The listing builds one solid part. Answer for the finished solid, in the listing's coordinates (mm). A direction names the side the tool comes from. Coordinates: 2 decimals unless noted, no trailing zeros. Loops run counter-clockwise (first coordinate to the right, second up) from the corner with the lowest first, then second, coordinate; pieces in that order, holes last. Notation, with made-up numbers: (14, 17) - (65, 17) arc R25 cw to (65, 51) - close; hole circle Ø5 at (17.25, 43.5). An arc over 180 degrees is marked (long way). Put each result on its own line as item: value.
```python
from build123d import *

# Parameters (mm, degrees)
SKETCH1_R           = 140
BOSS_EXTRUDE1_DEPTH = 3
CUT_EXTRUDE3_REACH  = 200.013
SKETCH19_R          = 1.5
CUT_EXTRUDE10_REACH = 200.013
SKETCH25_R          = 1.5
CUT_EXTRUDE4_REACH  = 200.013
FILLET2_R           = 10
SKETCH26_R          = 1.5
CUT_EXTRUDE11_DEPTH = 3
FILLET6_R           = 3
FILLET7_R           = 1


with BuildPart() as part:
    # Sketch1 → Boss-Extrude1 (new body)
    with BuildSketch(Plane(origin=(0, 0, 0), x_dir=(1, 0, 0), z_dir=(0, 1, 0))):
        with Locations(Location((0, 0, 0), (0, 0, 270))):
            Circle(SKETCH1_R)
    extrude(amount=BOSS_EXTRUDE1_DEPTH)

    # Sketch19 → Cut-Extrude3 (cut, up to next)
    with BuildSketch(Plane(origin=(0, 3, 0), x_dir=(1, 0, 0), z_dir=(0, 1, 0)), mode=Mode.PRIVATE) as cut_extrude3_sk1:
        with Locations(Location((-89.09545443, -67.882250994, 0), (0, 0, 270))):
            Circle(SKETCH19_R)
    cut_extrude3_tool1 = extrude(cut_extrude3_sk1.sketch, amount=-CUT_EXTRUDE3_REACH, mode=Mode.PRIVATE) & part.part
    # Sketch19 → Cut-Extrude3 (cut, up to next)
    with BuildSketch(Plane(origin=(0, 3, 0), x_dir=(1, 0, 0), z_dir=(0, 1, 0)), mode=Mode.PRIVATE) as cut_extrude3_sk2:
        with Locations(Location((-89.09545443, 67.882250994, 0), (0, 0, 270))):
            Circle(SKETCH19_R)
    cut_extrude3_tool2 = extrude(cut_extrude3_sk2.sketch, amount=-CUT_EXTRUDE3_REACH, mode=Mode.PRIVATE) & part.part
    # Sketch19 → Cut-Extrude3 (cut, up to next)
    with BuildSketch(Plane(origin=(0, 3, 0), x_dir=(1, 0, 0), z_dir=(0, 1, 0)), mode=Mode.PRIVATE) as cut_extrude3_sk3:
        with Locations(Location((89.09545443, 67.882250994, 0), (0, 0, 270))):
            Circle(SKETCH19_R)
    cut_extrude3_tool3 = extrude(cut_extrude3_sk3.sketch, amount=-CUT_EXTRUDE3_REACH, mode=Mode.PRIVATE) & part.part
    # Sketch19 → Cut-Extrude3 (cut, up to next)
    with BuildSketch(Plane(origin=(0, 3, 0), x_dir=(1, 0, 0), z_dir=(0, 1, 0)), mode=Mode.PRIVATE) as cut_extrude3_sk4:
        with Locations(Location((89.09545443, -67.882250994, 0), (0, 0, 270))):
            Circle(SKETCH19_R)
    cut_extrude3_tool4 = extrude(cut_extrude3_sk4.sketch, amount=-CUT_EXTRUDE3_REACH, mode=Mode.PRIVATE) & part.part
    # Sketch19 → Cut-Extrude3 (cut, up to next)
    with BuildSketch(Plane(origin=(0, 3, 0), x_dir=(1, 0, 0), z_dir=(0, 1, 0)), mode=Mode.PRIVATE) as cut_extrude3_sk5:
        with Locations(Location((-67.882250994, 89.09545443, 0), (0, 0, 270))):
            Circle(SKETCH19_R)
    cut_extrude3_tool5 = extrude(cut_extrude3_sk5.sketch, amount=-CUT_EXTRUDE3_REACH, mode=Mode.PRIVATE) & part.part
    # Sketch19 → Cut-Extrude3 (cut, up to next)
    with BuildSketch(Plane(origin=(0, 3, 0), x_dir=(1, 0, 0), z_dir=(0, 1, 0)), mode=Mode.PRIVATE) as cut_extrude3_sk6:
        with Locations(Location((67.882250994, 89.09545443, 0), (0, 0, 270))):
            Circle(SKETCH19_R)
    cut_extrude3_tool6 = extrude(cut_extrude3_sk6.sketch, amount=-CUT_EXTRUDE3_REACH, mode=Mode.PRIVATE) & part.part
    # Sketch19 → Cut-Extrude3 (cut, up to next)
    with BuildSketch(Plane(origin=(0, 3, 0), x_dir=(1, 0, 0), z_dir=(0, 1, 0)), mode=Mode.PRIVATE) as cut_extrude3_sk7:
        with Locations(Location((67.882250994, -89.09545443, 0), (0, 0, 270))):
            Circle(SKETCH19_R)
    cut_extrude3_tool7 = extrude(cut_extrude3_sk7.sketch, amount=-CUT_EXTRUDE3_REACH, mode=Mode.PRIVATE) & part.part
    # Sketch19 → Cut-Extrude3 (cut, up to next)
    with BuildSketch(Plane(origin=(0, 3, 0), x_dir=(1, 0, 0), z_dir=(0, 1, 0)), mode=Mode.PRIVATE) as cut_extrude3_sk8:
        with Locations(Location((-67.882250994, -89.09545443, 0), (0, 0, 270))):
            Circle(SKETCH19_R)
    cut_extrude3_tool8 = extrude(cut_extrude3_sk8.sketch, amount=-CUT_EXTRUDE3_REACH, mode=Mode.PRIVATE) & part.part
    add(cut_extrude3_tool1.solids().sort_by_distance((-89.095454, 3, 67.882251))[0], mode=Mode.SUBTRACT)
    add(cut_extrude3_tool2.solids().sort_by_distance((-89.095454, 3, -67.882251))[0], mode=Mode.SUBTRACT)
    add(cut_extrude3_tool3.solids().sort_by_distance((89.095454, 3, -67.882251))[0], mode=Mode.SUBTRACT)
    add(cut_extrude3_tool4.solids().sort_by_distance((89.095454, 3, 67.882251))[0], mode=Mode.SUBTRACT)
    add(cut_extrude3_tool5.solids().sort_by_distance((-67.882251, 3, -89.095454))[0], mode=Mode.SUBTRACT)
    add(cut_extrude3_tool6.solids().sort_by_distance((67.882251, 3, -89.095454))[0], mode=Mode.SUBTRACT)
    add(cut_extrude3_tool7.solids().sort_by_distance((67.882251, 3, 89.095454))[0], mode=Mode.SUBTRACT)
    add(cut_extrude3_tool8.solids().sort_by_distance((-67.882251, 3, 89.095454))[0], mode=Mode.SUBTRACT)

    # Sketch25 → Cut-Extrude10 (cut, up to next)
    with BuildSketch(Plane(origin=(0, 3, 0), x_dir=(1, 0, 0), z_dir=(0, 1, 0)), mode=Mode.PRIVATE) as cut_extrude10_sk1:
        with Locations(Location((-124, 50, 0), (0, 0, 270))):
            Circle(SKETCH25_R)
    cut_extrude10_tool1 = extrude(cut_extrude10_sk1.sketch, amount=-CUT_EXTRUDE10_REACH, mode=Mode.PRIVATE) & part.part
    # Sketch25 → Cut-Extrude10 (cut, up to next)
    with BuildSketch(Plane(origin=(0, 3, 0), x_dir=(1, 0, 0), z_dir=(0, 1, 0)), mode=Mode.PRIVATE) as cut_extrude10_sk2:
        with Locations(Location((-124, -50, 0), (0, 0, 270))):
            Circle(SKETCH25_R)
    cut_extrude10_tool2 = extrude(cut_extrude10_sk2.sketch, amount=-CUT_EXTRUDE10_REACH, mode=Mode.PRIVATE) & part.part
    add(cut_extrude10_tool1.solids().sort_by_distance((-124, 3, -50))[0], mode=Mode.SUBTRACT)
    add(cut_extrude10_tool2.solids().sort_by_distance((-124, 3, 50))[0], mode=Mode.SUBTRACT)

    # Sketch20 → Cut-Extrude4 (cut, up to next)
    with BuildSketch(Plane(origin=(0, 3, 0), x_dir=(1, 0, 0), z_dir=(0, 1, 0)), mode=Mode.PRIVATE) as cut_extrude4_sk1:
        Polygon((-553.578520829, 601.645168987), (-72, 120.066648158), (-50, 98.066648158), (50, 98.066648158), (72, 120.066648158), (553.578520829, 601.645168987), (553.578520829, 1963.754919995), (-553.578520829, 1963.754919995), align=None)
    cut_extrude4_tool1 = extrude(cut_extrude4_sk1.sketch, amount=-CUT_EXTRUDE4_REACH, mode=Mode.PRIVATE) & part.part
    add(cut_extrude4_tool1.solids().sort_by_distance((0, 3, -1137.970098))[0], mode=Mode.SUBTRACT)

    # Fillet2
    fillet2_edges = [part.edges().sort_by_distance(p)[0] for p in [
        (50, 1.5, -98.066648158),
        (-50, 1.5, -98.066648158),
    ]]
    fillet(fillet2_edges, radius=FILLET2_R)

    # Sketch26 → Cut-Extrude11 (cut)
    # profile 1 of 7: a face of its own
    with BuildSketch(Plane(origin=(0, 3, 0), x_dir=(1, 0, 0), z_dir=(0, 1, 0))):
        with BuildLine():
            Line((-79.056988797, -89.449340058), (-121.24355653, -70))
            ThreePointArc((-121.24355653, -70), (98.171098855, -99.812000028), (72, 120.066648158))
            Line((72, 120.066648158), (52.928932188, 100.995580347))
            ThreePointArc((52.928932188, 100.995580347), (49.6846987, 98.827852833), (45.857864376, 98.066648158))
            Line((45.857864376, 98.066648158), (-45.857864376, 98.066648158))
            ThreePointArc((-45.857864376, 98.066648158), (-49.6846987, 98.827852833), (-52.928932188, 100.995580347))
            Line((-52.928932188, 100.995580347), (-60.850013122, 108.91666128))
            ThreePointArc((-60.850013122, 108.91666128), (-75.23752201, 86.148205434), (-86.128818141, 61.515246573))
            Line((-86.128818141, 61.515246573), (-109.612709786, 69.893160276))
            ThreePointArc((-109.612709786, 69.893160276), (-124.799143171, 36.402937572), (-130, 0))
            ThreePointArc((-130, 0), (-125.518409602, -31.669231283), (-112.425579752, -60.851463362))
            Line((-112.425579752, -60.851463362), (-100.142136058, -66.514518839))
            Line((-100.142136058, -66.514518839), (-86.128818141, -61.515246573))
            ThreePointArc((-86.128818141, -61.515246573), (-81.664833416, -72.826250762), (-76.459826151, -83.815967535))
            Line((-76.459826151, -83.815967535), (-79.056988797, -89.449340058))
        make_face()
        with Locations((-67.882250994, -89.09545443)):
            Circle(SKETCH26_R, mode=Mode.SUBTRACT)
        with Locations((67.882250994, -89.09545443)):
            Circle(SKETCH26_R, mode=Mode.SUBTRACT)
        with Locations((89.09545443, -67.882250994)):
            Circle(SKETCH26_R, mode=Mode.SUBTRACT)
        with Locations((-67.882250994, 89.09545443)):
            Circle(SKETCH26_R, mode=Mode.SUBTRACT)
        with Locations((67.882250994, 89.09545443)):
            Circle(SKETCH26_R, mode=Mode.SUBTRACT)
        with Locations((89.09545443, 67.882250994)):
            Circle(SKETCH26_R, mode=Mode.SUBTRACT)
    # profile 2 of 7: a face of its own
    with BuildSketch(Plane(origin=(0, 3, 0), x_dir=(1, 0, 0), z_dir=(0, 1, 0))):
        with BuildLine():
            Line((-103.69839741, 78.400525346), (-88.170631715, 72.860971556))
            ThreePointArc((-88.170631715, 72.860971556), (-80.354415694, 89.303260425), (-70.993089828, 104.917602363))
            Line((-70.993089828, 104.917602363), (-73.383091495, 107.30760403))
            ThreePointArc((-73.383091495, 107.30760403), (-89.712698252, 94.083110983), (-103.69839741, 78.400525346))
        make_face()
    # profile 3 of 7: a face of its own
    with BuildSketch(Plane(origin=(0, 3, 0), x_dir=(1, 0, 0), z_dir=(0, 1, 0))):
        with Locations((-67.882250994, 89.09545443)):
            Circle(SKETCH26_R)
    # profile 4 of 7: a face of its own
    with BuildSketch(Plane(origin=(0, 3, 0), x_dir=(1, 0, 0), z_dir=(0, 1, 0))):
        with Locations(Location((-89.09545443, 67.882250994, 0), (0, 0, 270))):
            Circle(SKETCH26_R)
    # profile 5 of 7: a face of its own
    with BuildSketch(Plane(origin=(0, 3, 0), x_dir=(1, 0, 0), z_dir=(0, 1, 0))):
        with Locations(Location((-124, 50, 0), (0, 0, 270))):
            Circle(SKETCH26_R)
    # profile 6 of 7: a face of its own
    with BuildSketch(Plane(origin=(0, 3, 0), x_dir=(1, 0, 0), z_dir=(0, 1, 0))):
        with Locations(Location((-89.09545443, -67.882250994, 0), (0, 0, 270))):
            Circle(SKETCH26_R)
    # profile 7 of 7: a face of its own
    with BuildSketch(Plane(origin=(0, 3, 0), x_dir=(1, 0, 0), z_dir=(0, 1, 0))):
        with Locations(Location((-124, -50, 0), (0, 0, 270))):
            Circle(SKETCH26_R)
    extrude(amount=-CUT_EXTRUDE11_DEPTH, mode=Mode.SUBTRACT)

    # Fillet6
    fillet6_edges = [part.edges().sort_by_distance(p)[0] for p in [
        (-109.612709786, 1.5, -69.893160276),
        (-86.128818141, 1.5, -61.515246573),
        (-60.850013122, 1.5, -108.91666128),
        (-121.24355653, 1.5, 70),
        (-79.056988797, 1.5, 89.449340058),
        (-76.459826151, 1.5, 83.815967535),
        (-86.128818141, 1.5, 61.515246573),
        (-100.142136058, 1.5, 66.514518839),
        (-112.425579752, 1.5, 60.851463362),
        (-72, 1.5, -120.066648158),
        (-88.170631715, 1.5, -72.860971556),
        (-103.69839741, 1.5, -78.400525346),
    ]]
    fillet(fillet6_edges, radius=FILLET6_R)

    # Fillet7
    fillet7_edges = [part.edges().sort_by_distance(p)[0] for p in [
        (-73.383091495, 1.5, -107.30760403),
        (-70.993089828, 1.5, -104.917602363),
    ]]
    fillet(fillet7_edges, radius=FILLET7_R)


solid = part.part
```
1) Each of these flat-tipped pins is pushed along its axis until it touches: pin 1 (1.5 mm diameter, centred on x = -115, z = -54.5, fed in from +Y); pin 2 (1 mm diameter, centred on x = -70, y = 2.5, fed in from -Z); pin 3 (1 mm diameter, centred on y = 2, z = 57, fed in from -X). Where does it stop, or does it pass through?
Found:
pin 1: passes through
pin 2: stops at z = -118.55
pin 3: stops at x = -128.09
2) For faces 4 (the face through (-100.81, 1.52, 79.42)), 5 (the face through (-125.764, 1.521, 30.807)), 6 (the face through (-106.51, 1.52, 63.58)), determine the directions among +Z, -Z, +X, -X, +Y, -Y from which every point of the face is accessible in a straight line to the end or side of a thin tool.
Found:
face 4: +Z, -X, +Y, -Y
face 5: +X, +Y, -Y
face 6: +Y, -Y
3) Straight lines are drawn through the part: L1, parallel to Z at x = -92.5, y = 2.05; L2, parallel to Z at x = -94, y = 0.8; L3, parallel to X at y = 2.05, z = 50. For each, find the intervals that lie inside material, in ascending order. Write a range as [from, to].
Found:
L1: z = [-105.09, -91.34], [-74.41, -63.79], [63.79, 83.25]
L2: z = [-103.75, -89.8], [-74.94, -64.32], [64.32, 82.56]
L3: x = [-130.77, -125.5], [-122.5, -118.47]
4) For a pull along Z with two mould halves and no side action, classify faces 1 (the face through (-79.99, 1.52, -89.98)), 2 (the face through (-135.325, 1.479, -35.877)), 3 (the face through (-130, 3, -24)) as pulls with the +Z half, pulls with the -Z half, needs draft (parallel to the pull), parting line crosses it, or undercut.
Found:
face 1: undercut
face 2: parting line crosses it
face 3: needs draft
5) The part is cut by section A-A (x = -115.5). Give the vertices of the cut face in (y, z) (3 decimals), and give its area (3 significant figures).
Found:
outline: (0, -79.119) - (3, -79.119) - (3, -59.664) - (0, -59.664) - close; (0, 55.675) - (3, 55.675) - (3, 72.648) - (0, 72.648) - close
area: 109 mm^2
6) The part is cut by section B-B (y = 1.6). State how many separate pieces and enclosed holes the cut face has, and give its area (3 significant figures).
Found:
separate pieces: 1
enclosed holes: 5
area: 3,260 mm^2
7) The part is cut by section D-D (x = -104.5). Give the vertices of the cut face in (y, z), and give its area (3 significant figures).
Found:
outline: (0, -93.17) - (3, -93.17) - (3, -68.07) - (0, -68.07) - close; (0, 64.51) - (3, 64.51) - (3, 77.72) - (0, 77.72) - close
area: 115 mm^2
8) The part is cut by section C-C (z = 26). Give the vertices of the cut face in (x, y).
Found:
outline: (-137.56, 0) - (-127, 0) - (-127, 3) - (-137.56, 3) - close
